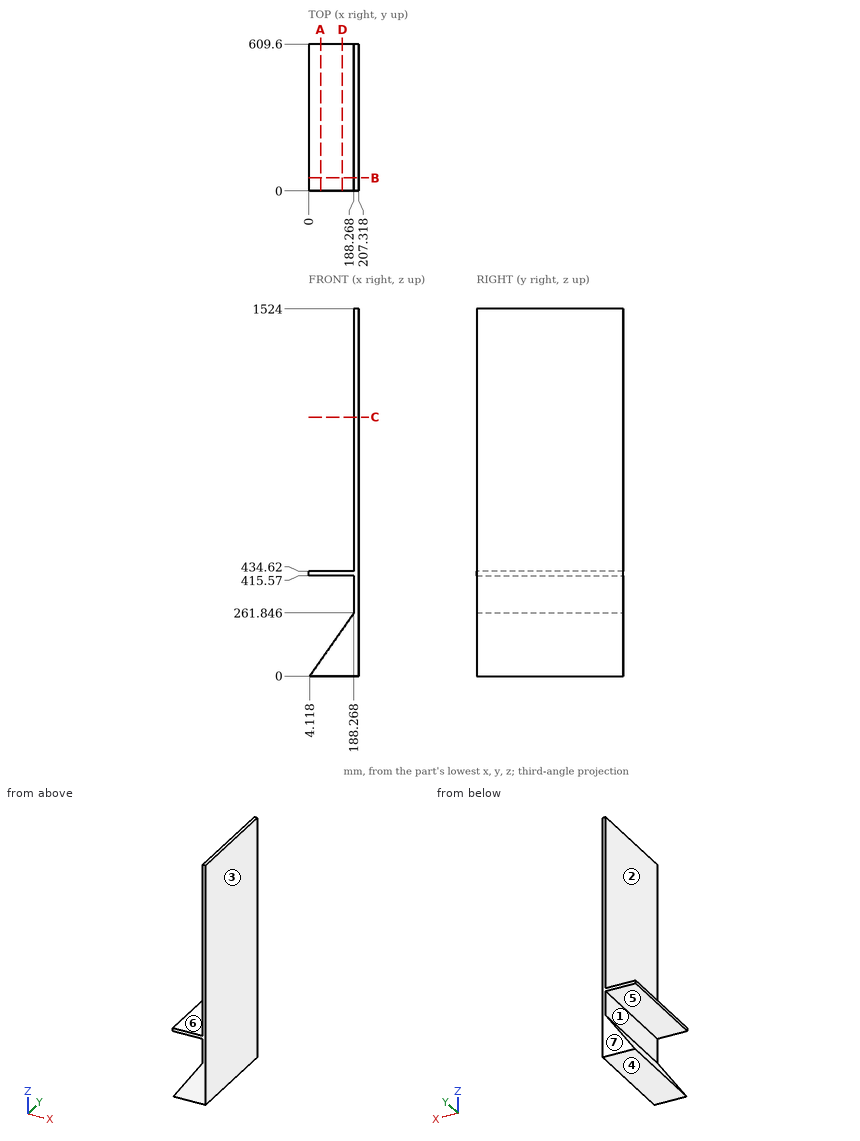
Study the drawing (mm; zero at the part's minimum x, y, z) and answer. A direction names the side the tool comes from. Give positions to 0.01 mm unless a question says otherwise; leave off trailing zeros. Loops run counter-clockwise (first coordinate to the right, second up) from the corner with the lowest first, then second, coordinate; pieces in that order, holes last. Notation, with made-up numbers: (60.5, -3.5) - (85.5, -3.5) arc R20 cw to (85.5, 21.5) - close; hole circle Ø7 at (24.25, -37). An arc over 180 degrees is marked (long way). Answer in a Markdown table with one row per item. Add a question column.
Q1. A tool of negligible diameter and unlimited length cuts with its end or side. For the marked faces 1, 2 and 3, from which of +Z, -Z, +X, -X, +Y, -Y can it reach the whole face along a straight path? Write none if from no direction.
Q2. Determine the mould class of the marked faces 4, 5, 6 and 7 for opening direction Z: released by +Z, released by -Z, zero draft, split by the parting line, or undercut.
Q3. Consider line 1 along X through (y, z) = (439, 1150.5); line 2 along Z through (x, y) = (121.5, 285) (1 decimal); line 3 along Z through (x, y) = (180, 390). Determine where each line is inside the solid, lowest interval first.
Q4. The part is cut by section A-A (x = 50). Determine the outline of the cut face in (y, z), and give its area (3 significant figures).
Q5. Each of these flat-tipped pins is pushed along its axis until it touches: P1, Ø3, axis at y = 181, z = 292.5, coming from the -X side; P2, Ø1, axis at x = 55, y = 317, coming from the +Z side. Where does it stop, or does it pass through?
Q6. The part is cut by section D-D (x = 140.5). Determine the outline of the cut face in (y, z).
Q7. The part is cut by section B-B (y = 53.5). Determine the outline of the cut face in (x, z), and give its area (3 significant figures).
Q8. The part is cut by section C-C (z = 1075). Determine the outline of the cut face in (x, y), and give its area (3 significant figures).
Solution:
| question | item | result |
|---|---|---|
| 1 | face 1 | -X, +Y, -Y |
| 1 | face 2 | +Z, -X, +Y, -Y |
| 1 | face 3 | +Z, -Z, +X, +Y, -Y |
| 2 | face 4 | released by -Z |
| 2 | face 5 | undercut |
| 2 | face 6 | released by +Z |
| 2 | face 7 | zero draft |
| 3 | line 1 | x = 188.27 to 207.32 |
| 3 | line 2 | z = 0 to 166.9, 415.6 to 434.6 |
| 3 | line 3 | z = 0 to 250.09, 415.57 to 434.62 |
| 4 | outline | (0, 0) - (609.6, 0) - (609.6, 65.24) - (0, 65.24) - close; (0, 415.57) - (609.6, 415.57) - (609.6, 434.62) - (0, 434.62) - close |
| 4 | area | 51,400 mm² |
| 5 | P1 | stops at x = 188.27 |
| 5 | P2 | stops at z = 434.62 |
| 6 | outline | (0, 0) - (609.6, 0) - (609.6, 193.92) - (0, 193.92) - close; (0, 415.57) - (609.6, 415.57) - (609.6, 434.62) - (0, 434.62) - close |
| 7 | outline | (0, 415.57) - (188.27, 415.57) - (188.27, 261.85) - (4.12, 0) - (207.32, 0) - (207.32, 1524) - (188.27, 1524) - (188.27, 434.62) - (0, 434.62) - close |
| 7 | area | 56,700 mm² |
| 8 | outline | (188.27, 0) - (207.32, 0) - (207.32, 609.6) - (188.27, 609.6) - close |
| 8 | area | 11,600 mm² |
